Work out the finished part from the listing and answer in its coordinate system (mm). A direction names the side the tool comes from. Round coordinates to 2 decimals unless told otherwise and drop trailing zeros. Order: outer loops, then holes, each group sorted by start corner. A loop starts at its lowest first (then second) coordinate and runs counter-clockwise, first axis right, second up. Notation, with made-up numbers: (23, 36.25) -> (55, 36.25) arc R25 ccw to (55, 60.25) -> close; hole circle Ø3 at (26, 74.5). An arc over 180 degrees is marked (long way). Use one line per item in the form item = value.
```python
from build123d import *

# Parameters (mm, degrees)
SKETCH1_W           = 39
SKETCH1_H           = 39
SKETCH1_R           = 3.25
BOSS_EXTRUDE1_DEPTH = 10
SKETCH2_W           = 64
SKETCH2_H           = 58
SKETCH2_R           = 3.25
BOSS_EXTRUDE2_DEPTH = 5
BOSS_EXTRUDE3_REACH = 88.817
SKETCH3_W           = 10
SKETCH3_H           = 48
SKETCH5_W           = 39
SKETCH5_H           = 25
SKETCH5_R           = 3.25
BOSS_EXTRUDE4_DEPTH = 10


with BuildPart() as part:
    # Sketch1 → Boss-Extrude1 (new body)
    with BuildSketch(Plane(origin=(0, 0, 0), x_dir=(1, 0, 0), z_dir=(0, 1, 0))):
        with Locations((19.5, 19.5)):
            Rectangle(SKETCH1_W, SKETCH1_H)
        with Locations(Location((7, 32, 0), (0, 0, 270))):
            Circle(SKETCH1_R, mode=Mode.SUBTRACT)
        with Locations(Location((32, 32, 0), (0, 0, 270))):
            Circle(SKETCH1_R, mode=Mode.SUBTRACT)
        with Locations(Location((32, 7, 0), (0, 0, 270))):
            Circle(SKETCH1_R, mode=Mode.SUBTRACT)
        with Locations(Location((7, 7, 0), (0, 0, 270))):
            Circle(SKETCH1_R, mode=Mode.SUBTRACT)
    extrude(amount=BOSS_EXTRUDE1_DEPTH)

    # Sketch2 → Boss-Extrude2 (add, symmetric)
    with BuildSketch(Plane.XY.offset(-19.5)):
        with Locations((19.5, 29)):
            Rectangle(SKETCH2_W, SKETCH2_H)
        with Locations((-5.5, 51)):
            Circle(SKETCH2_R, mode=Mode.SUBTRACT)
        with Locations((44.5, 51)):
            Circle(SKETCH2_R, mode=Mode.SUBTRACT)
        with Locations((-5.5, 24)):
            Circle(SKETCH2_R, mode=Mode.SUBTRACT)
        with Locations((44.5, 24)):
            Circle(SKETCH2_R, mode=Mode.SUBTRACT)
    extrude(amount=BOSS_EXTRUDE2_DEPTH, both=True)

    # Sketch3 → Boss-Extrude3 (add, up to next)
    with BuildSketch(Plane.XY, mode=Mode.PRIVATE) as boss_extrude3_sk1:
        with Locations((19.5, 34)):
            Rectangle(SKETCH3_W, SKETCH3_H)
    boss_extrude3_tool1 = extrude(boss_extrude3_sk1.sketch, amount=-BOSS_EXTRUDE3_REACH, mode=Mode.PRIVATE) - part.part
    add(boss_extrude3_tool1.solids().sort_by_distance((19.5, 34, 0))[0])

    # Sketch5 → Boss-Extrude4 (add)
    with BuildSketch(Plane(origin=(0, 10, 0), x_dir=(1, 0, 0), z_dir=(0, 1, 0))):
        with Locations((19.5, 51.5)):
            Rectangle(SKETCH5_W, SKETCH5_H)
        with Locations(Location((7, 57, 0), (0, 0, 270))):
            Circle(SKETCH5_R, mode=Mode.SUBTRACT)
        with Locations(Location((32, 57, 0), (0, 0, 270))):
            Circle(SKETCH5_R, mode=Mode.SUBTRACT)
    extrude(amount=-BOSS_EXTRUDE4_DEPTH)


solid = part.part
```
Item 1: For faces 5 (the flat face through (28, 10, -7)), 6 (the flat face through (14.5, 34, -7)), 7 (the flat face through (39, 5, -7)), determine the directions among +Z, -Z, +X, -X, +Y, -Y from which every point of the face is accessible in a straight line to the end or side of a thin tool.
Findings:
face_5 = +Z, +X, +Y
face_6 = +Z, -X, +Y
face_7 = +Z, +X, +Y, -Y
Item 2: The part is cut by section A-A, the plane y = 4.5. Give the vertices of the cut face in (x, z).
Findings:
outline = (-12.5, -24.5) -> (0, -24.5) -> (0, -64) -> (39, -64) -> (39, -24.5) -> (51.5, -24.5) -> (51.5, -14.5) -> (39, -14.5) -> (39, 0) -> (0, 0) -> (0, -14.5) -> (-12.5, -14.5) -> close; hole circle Ø6.5 at (7, -57); hole circle Ø6.5 at (7, -32); hole circle Ø6.5 at (7, -7); hole circle Ø6.5 at (32, -57); hole circle Ø6.5 at (32, -32); hole circle Ø6.5 at (32, -7)
Item 3: Flat-ended cylindrical pins translate along their axes: P1, Ø7.5, axis at x = -5.5, y = 24, coming from the +Z side; P2, Ø11, axis at y = 7, z = -44.5, coming from the -X side; P3, Ø10.5, axis at x = 7, z = -57, coming from the +Y side. Find the tip coordinate at first contact, or state that the pin passes through.
Findings:
P1 = -14.5
P2 = 0
P3 = 10
Item 4: The part is cut by section C-C, the plane z = -7. Give the vertices of the cut face in (x, y).
Findings:
outline = (0, 0) -> (3.75, 0) -> (3.75, 10) -> (0, 10) -> close; (10.25, 0) -> (28.75, 0) -> (28.75, 10) -> (24.5, 10) -> (24.5, 58) -> (14.5, 58) -> (14.5, 10) -> (10.25, 10) -> close; (35.25, 0) -> (39, 0) -> (39, 10) -> (35.25, 10) -> close
Item 5: Determine the mould class of faces 1 (the flat face through (0, 5, -44)), 2 (the cylindrical face through (7.143, 5.07, -60.247)), 3 (the flat face through (19, 0, -32)), 4 (the flat face through (39, 5, -44)) for opening direction X: released by +X, released by -X, zero draft, split by the parting line, or undercut.
Findings:
face_1 = released by -X
face_2 = undercut
face_3 = zero draft
face_4 = released by +X
Item 6: Consider line 1 along Y through (x, z) = (-5.5, -20); line 2 along X through (y, z) = (5, -32); line 3 along Z through (x, y) = (34, 47). Determine where each line is inside the solid, lowest interval first.
Findings:
line_1 = 0 to 20.75, 27.25 to 47.75, 54.25 to 58
line_2 = 0 to 3.75, 10.25 to 28.75, 35.25 to 39
line_3 = -24.5 to -14.5
Item 7: The part is cut by section B-B, the plane x = 32. Give the vertices of the cut face in (y, z), and give its area (3 significant figures).
Findings:
outline = (0, -64) -> (10, -64) -> (10, -60.25) -> (0, -60.25) -> close; (0, -53.75) -> (10, -53.75) -> (10, -35.25) -> (0, -35.25) -> close; (0, -28.75) -> (10, -28.75) -> (10, -24.5) -> (58, -24.5) -> (58, -14.5) -> (10, -14.5) -> (10, -10.25) -> (0, -10.25) -> close; (0, -3.75) -> (10, -3.75) -> (10, 0) -> (0, 0) -> close
area = 925 mm^2
Item 8: The part is cut by section D-D, the plane y = 51. Give the vertices of the cut face in (x, z).
Findings:
outline = (-12.5, -24.5) -> (-8.75, -24.5) -> (-8.75, -14.5) -> (-12.5, -14.5) -> close; (-2.25, -24.5) -> (41.25, -24.5) -> (41.25, -14.5) -> (24.5, -14.5) -> (24.5, 0) -> (14.5, 0) -> (14.5, -14.5) -> (-2.25, -14.5) -> close; (47.75, -24.5) -> (51.5, -24.5) -> (51.5, -14.5) -> (47.75, -14.5) -> close
